Verification items for this drawing (mm, ordinates from the low corner). A direction names the side the tool comes from. Round coordinates to 2 decimals unless told otherwise and drop trailing zeros. Loops run counter-clockwise (first coordinate to the right, second up) from the corner with the lowest first, then second, coordinate; pieces in that order, holes last. Notation, with made-up numbers: M -13.75,53 L -6.75,53 A14 ccw -6.75,59 Z; hole C -12.5,11 d1. An arc over 180 degrees is marked long. Answer as CSV lines item,"result".
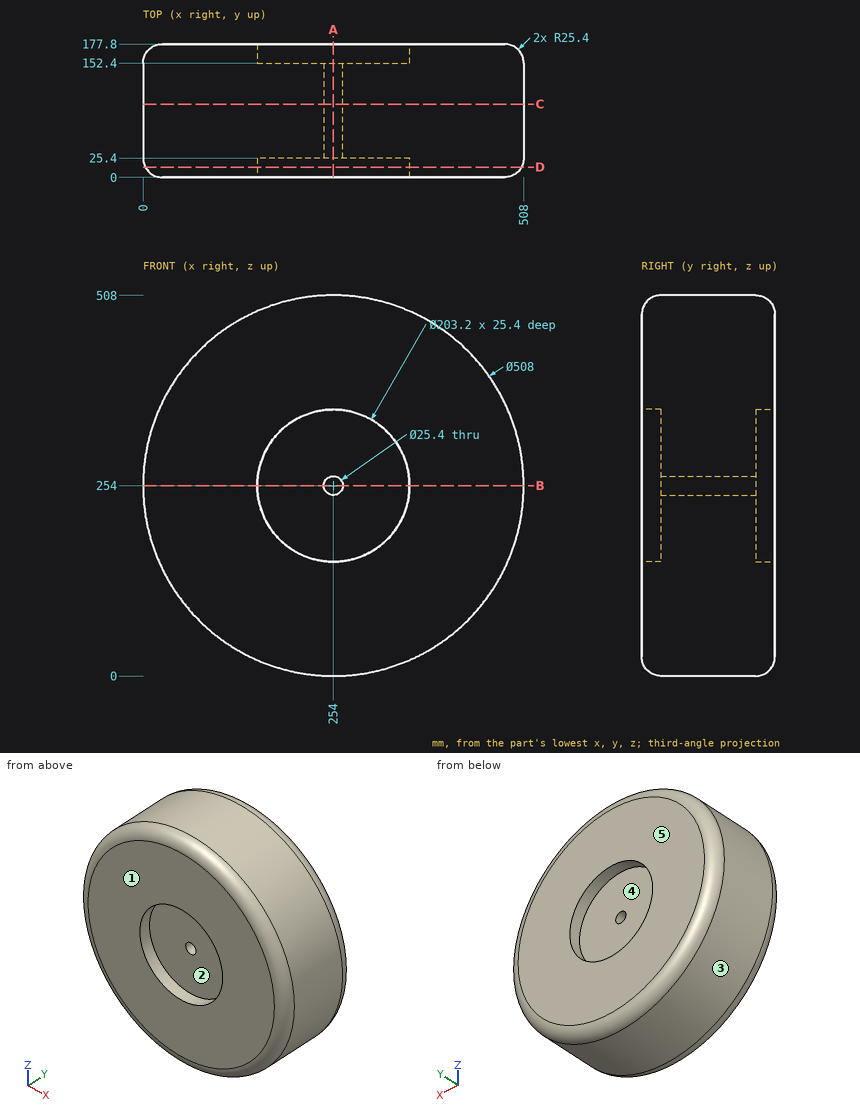
1) Go/stop test with flat-tipped pins: pin 1 (1.5 mm diameter, centred on x = 377, y = 66, fed in from -Z); pin 2 (2 mm diameter, centred on x = 420.5, y = 90.5, fed in from -Z); pin 3 (10 mm diameter, centred on x = 105.5, y = 52, fed in from -Z); pin 4 (1.5 mm diameter, centred on x = 185.5, z = 143, fed in from -Y). Record where each tip stops, or that it passes through.
Here are the results:
pin 1,"stops at z = 31.35"
pin 2,"stops at z = 61.32"
pin 3,"stops at z = 44.42"
pin 4,"stops at y = 0"
2) Material ranges on probe 1 along Z at (x, y) = (254, 123); probe 2 along Z at (x, y) = (254, 7); probe 3 along Y at (x, z) = (302, 314.5), recorded low to high.
Here are the results:
probe 1,"z = 0 to 241.3, 266.7 to 508"
probe 2,"z = 7.89 to 152.4, 355.6 to 500.11"
probe 3,"y = 25.4 to 152.4"
3) Section check A-A (x = 254). Record the cut outline in (y, z).
Here are the results:
outline,"M 0,25.4 A25.4 ccw 25.4,0 L 152.4,0 A25.4 ccw 177.8,25.4 L 177.8,152.4 L 152.4,152.4 L 152.4,241.3 L 25.4,241.3 L 25.4,152.4 L 0,152.4 Z; M 0,355.6 L 25.4,355.6 L 25.4,266.7 L 152.4,266.7 L 152.4,355.6 L 177.8,355.6 L 177.8,482.6 A25.4 ccw 152.4,508 L 25.4,508 A25.4 ccw 0,482.6 Z"
4) Draft check along X on the marked faces 3, 4 and 5. Enter one of: +X half, -X half, draft (parallel to the pull), parting line (faces both ways), or undercut.
Here are the results:
face 3,"parting line"
face 4,"undercut"
face 5,"draft"
5) Section check C-C (y = 97.5). Record the cut outline in (x, z).
Here are the results:
outline,"C 254,254 d508; hole C 254,254 d25.4"
6) Set-up check for the marked faces 1 and 2: record each of +Z, -Z, +X, -X, +Y, -Y from which the full face is reachable in a straight line by a thin tool's end or side.
Here are the results:
face 1,"+Z, -Z, +X, -X, -Y"
face 2,"-Y"
7) Section check D-D (y = 13.5). Record the cut outline in (x, z).
Here are the results:
outline,"C 254,254 d502.08; hole C 254,254 d203.2"
8) Section check B-B (z = 254). Record the cut outline in (x, y), plus the area to 3 significant figures.
Here are the results:
outline,"M 0,25.4 A25.4 ccw 25.4,0 L 152.4,0 L 152.4,25.4 L 241.3,25.4 L 241.3,152.4 L 152.4,152.4 L 152.4,177.8 L 25.4,177.8 A25.4 ccw 0,152.4 Z; M 266.7,25.4 L 355.6,25.4 L 355.6,0 L 482.6,0 A25.4 ccw 508,25.4 L 508,152.4 A25.4 ccw 482.6,177.8 L 355.6,177.8 L 355.6,152.4 L 266.7,152.4 Z"
area,"76,200 mm^2"
